Design review of the part shown in the three views and the two pictorial views. Dimensions are in mm from the part's minimum x, y and z. A direction names the side the tool comes from. Give positions to 0.01 mm unless a question says otherwise; leave off trailing zeros. Order: outer loops, then holes, each group sorted by start corner. A loop starts at its lowest first (then second) coordinate and runs counter-clockwise, first axis right, second up.
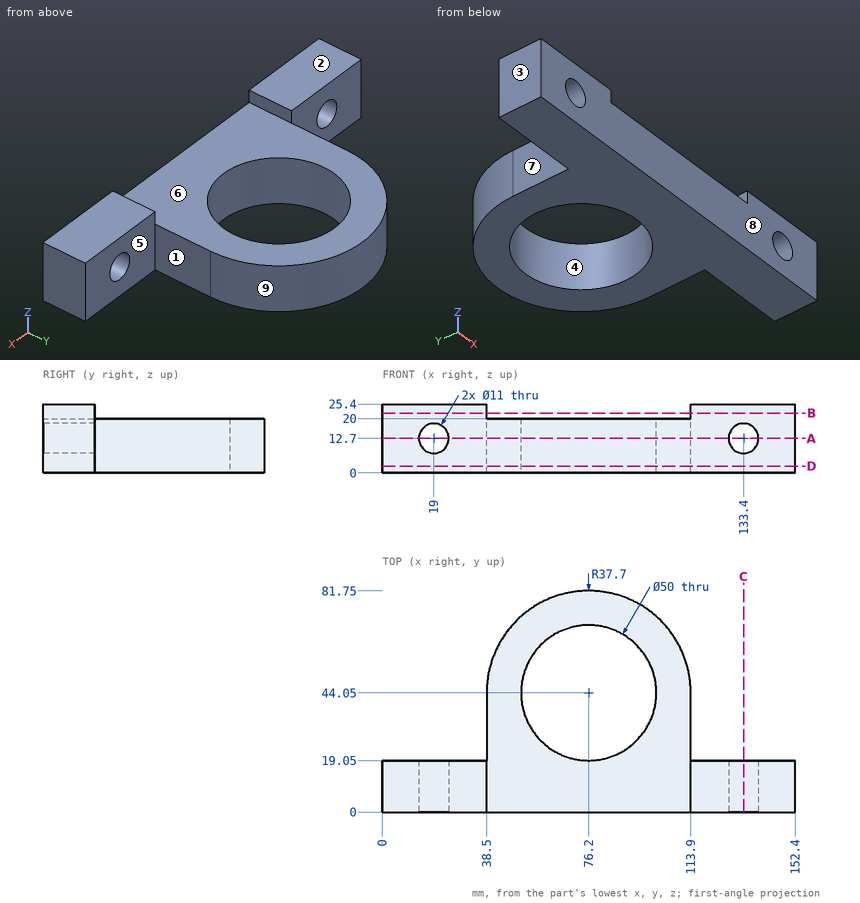
Item 1: Take a section at C-C (x = 133.4). Give the boundary of the cut face in (y, z).
Values found:
outline: (0, 0) - (19.05, 0) - (19.05, 7.2) - (0, 7.2) - close; (0, 18.2) - (19.05, 18.2) - (19.05, 25.4) - (0, 25.4) - close
Item 2: For the marked faces 5, 6, 7, 8 and 9, list the 3-axis set-ups (+Z, -Z, +X, -X, +Y, -Y) from which the entire face can be reached by the end or side of a thin tool; tool diameter is ignored.
Values found:
face 5: +Z, -Z, +X, +Y
face 6: +Z, +Y, -Y
face 7: +Z, -Z, -X, +Y
face 8: +Z, -Z, +X, -X, -Y
face 9: +Z, -Z, +Y
Item 3: Draft analysis for pull direction X (two halves, no side actions). For the marked faces 1, 2, 3 and 4, state which applies: released by +X, released by -X, zero draft, split by the parting line, or undercut.
Values found:
face 1: released by +X
face 2: zero draft
face 3: released by -X
face 4: undercut
Item 4: Take a section at B-B (z = 22). Give the boundary of the cut face in (x, y), and give its area (3 significant figures).
Values found:
outline: (0, 0) - (38.5, 0) - (38.5, 19.05) - (0, 19.05) - close; (113.9, 0) - (152.4, 0) - (152.4, 19.05) - (113.9, 19.05) - close
area: 1,470 mm2
Item 5: Clearance check with flat-ended pins moving along their axes: pin 1 Ø2.5 at (y, z) = (11.5, 21.5) entering from -X; pin 2 Ø4 at (y, z) = (28, 9) entering from -X; pin 3 Ø12.5 at (x, z) = (126, 11) entering from +Y; pin 4 Ø3 at (y, z) = (32.5, 18) entering from +X. State where each tip first meets the part, or that it passes through.
Values found:
pin 1: stops at x = 0
pin 2: stops at x = 38.5
pin 3: stops at y = 19.05
pin 4: stops at x = 113.9
Item 6: Take a section at D-D (z = 2.5). Give the boundary of the cut face in (x, y), and give its area (3 significant figures).
Values found:
outline: (0, 0) - (152.4, 0) - (152.4, 19.05) - (113.9, 19.05) - (113.9, 44.05) arc R37.7 ccw to (38.5, 44.05) - (38.5, 19.05) - (0, 19.05) - close; hole circle Ø50 at (76.2, 44.05)
area: 5,060 mm2
Item 7: For line 1 (X direction, y = 7, z = 7.75); line 2 (Z direction, x = 133.4, y = 13.5); line 3 (Y direction, x = 25.5, z = 3), list the stretches that pass through material, from the lowest coordinate up.
Values found:
line 1: x = 0 to 16.6, 21.4 to 131, 135.8 to 152.4
line 2: z = 0 to 7.2, 18.2 to 25.4
line 3: y = 0 to 19.05
Item 8: Take a section at A-A (z = 12.7). Give the boundary of the cut face in (x, y).
Values found:
outline: (0, 0) - (13.5, 0) - (13.5, 19.05) - (0, 19.05) - close; (24.5, 0) - (127.9, 0) - (127.9, 19.05) - (113.9, 19.05) - (113.9, 44.05) arc R37.7 ccw to (38.5, 44.05) - (38.5, 19.05) - (24.5, 19.05) - close; (138.9, 0) - (152.4, 0) - (152.4, 19.05) - (138.9, 19.05) - close; hole circle Ø50 at (76.2, 44.05)
